```python
from build123d import *


with BuildPart() as part:
    # 草图1 → Cable_gland_section (revolve)
    with BuildSketch(Plane.XY, mode=Mode.PRIVATE) as cable_gland_section_sk:
        Polygon((3.2, 0), (6.5, 0), (6.5, 6), (7, 6), (7, 9), (9, 9), (9, 10), (3.2, 10), align=None)
    revolve(cable_gland_section_sk.sketch.rotate(Axis((0, 0, 0), (0, 1, 0)), 90), axis=Axis((0, 0, 0), (0, 1, 0)))


solid = part.part
```
Verification items for the finished model (mm, model axes). A direction names the side the tool comes from. Give positions to 0.01 mm unless a question says otherwise; leave off trailing zeros. Loops run counter-clockwise (first coordinate to the right, second up) from the corner with the lowest first, then second, coordinate; pieces in that order, holes last. Notation, with made-up numbers: M -38.5,60 L -6.5,60 A20 ccw -6.5,98 Z; hole C 0,-26 d7. An arc over 180 degrees is marked long. Return JSON: item names as keys, results as strings.
1) Section check B-B, the plane z = 0. Enter the section's corners in (x, y), and give its area (3 significant figures).
Findings:
{"outline": "M -9,9 L -7,9 L -7,6 L -6.5,6 L -6.5,0 L -3.2,0 L -3.2,10 L -9,10 Z; M 3.2,0 L 6.5,0 L 6.5,6 L 7,6 L 7,9 L 9,9 L 9,10 L 3.2,10 Z", "area": "74.0 mm2"}
2) Material ranges on L1, parallel to X at y = 6.5, z = 0; L2, parallel to X at y = 2.5, z = 0; L3, parallel to Y at x = -6.5, z = -1, recorded low to high. Write a range as [from, to].
Findings:
{"L1": "x = [-7, -3.2], [3.2, 7]", "L2": "x = [-6.5, -3.2], [3.2, 6.5]", "L3": "y = [6, 10]"}
3) Gauge pin test, flat ends, axial feed: P1, Ø5, axis at x = -1, y = 5, coming from the -Z side; P2, Ø1, axis at x = -4, y = 1.5, coming from the +Z side; P3, Ø4, axis at y = 2.5, z = 7, coming from the +X side. Record the tip position at first contact, or that the pin passes through.
Findings:
{"P1": "stops at z = -7", "P2": "stops at z = 5.48", "P3": "stops at x = 4.15"}
4) Section check D-D, the plane x = -5.25. Enter the section's corners in (y, z).
Findings:
{"outline": "M 0,-3.83 L 6,-3.83 L 6,-4.63 L 9,-4.63 L 9,-7.31 L 10,-7.31 L 10,7.31 L 9,7.31 L 9,4.63 L 6,4.63 L 6,3.83 L 0,3.83 Z"}
5) Section check C-C, the plane y = 5.5. Enter the section's corners in (x, z), and give its area (3 significant figures).
Findings:
{"outline": "C 0,0 d13; hole C 0,0 d6.4", "area": "101 mm2"}
6) Mould release check, pull along Z, two halves, no side actions. Record for faces 1 (the cylindrical face through (3.955, 3.042, 5.158)), 2 (the cylindrical face through (-0.961, 4.93, -3.052)), 3 (the flat face through (4, 10, 0)): released by +Z, released by -Z, zero draft, split by the parting line, or undercut.
Findings:
{"face 1": "split by the parting line", "face 2": "undercut", "face 3": "zero draft"}
7) Tool access check on faces 4 (the flat face through (-2, 0, -3)), 5 (the flat face through (7.3, 9, 0)). Record the directions out of +Z, -Z, +X, -X, +Y, -Y that give a thin tool (end or side, any length) a straight path to the whole face; none if there is none.
Findings:
{"face 4": "+Z, -Z, +X, -X, -Y", "face 5": "-Y"}
8) Section check A-A, the plane x = 0. Enter the section's corners in (y, z), and give its area (3 significant figures).
Findings:
{"outline": "M 0,-6.5 L 6,-6.5 L 6,-7 L 9,-7 L 9,-9 L 10,-9 L 10,-3.2 L 0,-3.2 Z; M 0,3.2 L 10,3.2 L 10,9 L 9,9 L 9,7 L 6,7 L 6,6.5 L 0,6.5 Z", "area": "74.0 mm2"}
